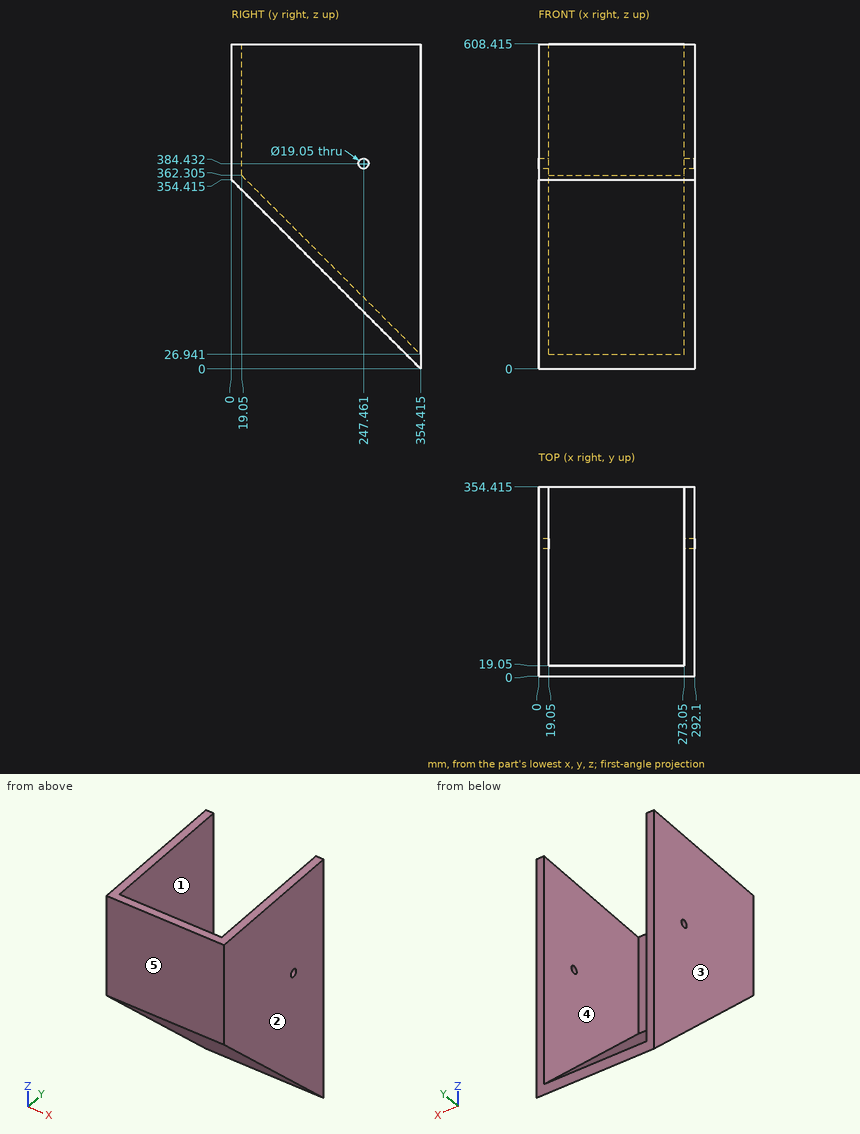
Design review of the part shown in the three views and the two pictorial views. Dimensions are in mm from the part's minimum x, y and z. A direction names the side the tool comes from. Coordinates: 2 decimals unless noted, no trailing zeros.
1) To check wall thickness, follow probe 1 along X at (y, z) = (47.5, 579.5); probe 2 along Y at (x, z) = (62, 568.5). State the ranges of each line that lie inside material, in increasing order.
2) The part is to be moulded in two halves that separate along X. For the marked faces 3, 4 and 5, say which applies: pulls with the +X half, pulls with the -X half, needs draft (parallel to the pull), parting line crosses it, or undercut.
3) Clearance check with flat-ended pins moving along their axes: pin 1 Ø10 at (x, z) = (126, 229.5) entering from -Y (1 decimal); pin 2 Ø12 at (x, y) = (239, 227) entering from +Z (1 decimal); pin 3 Ø4 at (x, z) = (134, 373.5) entering from +Y. State where each tip first meets the part, or that it passes through.
4) Machinability: for the marked faces 1 and 2, which of the approach directions +Z, -Z, +X, -X, +Y, -Y give a long, thin tool a straight path to every point of the face, cutting with its end or side? Answer none if there is none.
Answer list:
1. probe 1: x = 0 to 19.05, 273.05 to 292.1
1. probe 2: y = 0 to 19.05
2. face 3: pulls with the -X half
2. face 4: undercut
2. face 5: needs draft
3. pin 1: stops at y = 119.9
3. pin 2: stops at z = 160.4
3. pin 3: stops at y = 19.05
4. face 1: +Z, +Y
4. face 2: +Z, -Z, +X, +Y, -Y
